```python
from build123d import *

# Parameters (mm, degrees)
F0_W        = 57.15
F0_H        = 50.8
F1_DEPTH    = 6.35
F2_W        = 13.208
F2_H        = 1.190625
F3_DEPTH    = 50.801
F4_SIZE     = 5.08
F5_W        = 3.4
F5_H        = 15
F6_DEPTH    = 18
F7_W        = 13.208
F7_H        = 1.5875
F8_DEPTH    = 57.151
F9_T1_DEPTH = 13.208
F9_T3_DEPTH = 13.208
F11_D       = 5
F12_DEPTH   = 36.676


# Not quite as in the source:
# - a fillet or chamfer that OpenCascade refuses, or shapes differently, is made with other operations: its cross-section is extruded or revolved along the edge and cut away or added


with BuildPart() as f1:
    # F0 (on Top) → F1 (new body)
    with BuildSketch(Plane.XY):
        Rectangle(F0_W, F0_H)
    extrude(amount=F1_DEPTH)

    # F2 (on face) → F3 (cut, through all)
    with BuildSketch(Plane.XZ.offset(25.4)):
        with Locations((-16.129, 5.7546875)):
            Rectangle(F2_W, F2_H)
        with Locations((16.129, 5.7546875)):
            Rectangle(F2_W, F2_H)
    extrude(amount=-F3_DEPTH, mode=Mode.SUBTRACT)

    # F4
    f4_edges = [f1.edges().sort_by_distance(p)[0] for p in [
        (-16.129, -25.4, 5.159375),
        (16.129, -25.4, 5.159375),
        (-16.129, 25.4, 5.159375),
        (16.129, 25.4, 5.159375),
    ]]
    chamfer(f4_edges, length=F4_SIZE)

    # F5 (on face) → F6 (join)
    with BuildSketch(Plane.XY.offset(6.35)):
        Rectangle(F5_W, F5_H)
        with Locations((6.4, 0)):
            Rectangle(F5_W, F5_H)
        with Locations((-6.4, 0)):
            Rectangle(F5_W, F5_H)
    extrude(amount=F6_DEPTH)

    # F7 (on face) → F8 (cut, through all)
    with BuildSketch(Plane.YZ.offset(28.575)):
        with Locations((-16.129, 5.55625)):
            Rectangle(F7_W, F7_H)
        with Locations((16.129, 5.55625)):
            Rectangle(F7_W, F7_H)
    extrude(amount=-F8_DEPTH, mode=Mode.SUBTRACT)

    # F9: chamfer of 5.08 on 4 edges, made by hand

    # F9_s2 → F9_t1 (cut)
    with BuildSketch(Plane.XZ.offset(-22.733)):
        Polygon((28.575, -0.3175), (23.495, 4.7625), (28.575, 4.7625), align=None)
        Polygon((-28.575, -0.3175), (-23.495, 4.7625), (-28.575, 4.7625), align=None)
    extrude(amount=F9_T1_DEPTH, mode=Mode.SUBTRACT)

    # F9_s4 → F9_t3 (cut)
    with BuildSketch(Plane.XZ.offset(9.525)):
        Polygon((28.575, -0.3175), (23.495, 4.7625), (28.575, 4.7625), align=None)
        Polygon((-28.575, -0.3175), (-23.495, 4.7625), (-28.575, 4.7625), align=None)
    extrude(amount=F9_T3_DEPTH, mode=Mode.SUBTRACT)

    # F11 (through all)
    with Locations(Plane.YZ.offset(8.1)):
        with Locations((0, 16.85)):
            Hole(F11_D / 2)

    # F10 (on face) → F12 (cut, through all)
    with BuildSketch(Plane.YZ.offset(8.1)):
        with BuildLine():
            Line((-7.5, 24.35), (-7.5, 16.85))
            ThreePointArc((-7.5, 16.85), (-5.3033008589, 22.1533008589), (0, 24.35))
            Line((0, 24.35), (-7.5, 24.35))
        make_face()
        with BuildLine():
            Line((7.5, 24.35), (0, 24.35))
            ThreePointArc((0, 24.35), (5.3033008589, 22.1533008589), (7.5, 16.85))
            Line((7.5, 16.85), (7.5, 24.35))
        make_face()
    extrude(amount=-F12_DEPTH, mode=Mode.SUBTRACT)


solid = f1.part
```
Geometry: final body of the model. Coordinates: model frame, mm. A direction names the side the tool comes from. Round coordinates to 2 decimals unless told otherwise and drop trailing zeros. Order: outer loops, then holes, each group sorted by start corner. A loop starts at its lowest first (then second) coordinate and runs counter-clockwise, first axis right, second up. Notation, with made-up numbers: M 64.25,3 L 122.25,3 A7 cw 122.25,8 Z; hole C 29,28.25 d2. An arc over 180 degrees is marked long. One line per item, written item: value.
(1) Pin query (flat end, axial travel): P1, Ø3, axis at x = -5, z = 19.5, coming from the +Y side; P2, Ø12, axis at y = 0, z = 14.5, coming from the +X side; P3, Ø4, axis at x = -15, y = -0.5, coming from the +Z side. Return the tip coordinate at first contact, or that it passes through.
Result sheet:
P1: y = 7.41
P2: x = 8.1
P3: z = 5.16
(2) Cut plane B-B (z = 9). Return the cut outline in (x, y).
Result sheet:
outline: M -8.1,-7.5 L -4.7,-7.5 L -4.7,7.5 L -8.1,7.5 Z; M -1.7,-7.5 L 1.7,-7.5 L 1.7,7.5 L -1.7,7.5 Z; M 4.7,-7.5 L 8.1,-7.5 L 8.1,7.5 L 4.7,7.5 Z
(3) Cut plane C-C (y = -6). Return the cut outline in (x, z) (3 decimals).
Result sheet:
outline: M -28.575,0 L 28.575,0 L 28.575,6.35 L 22.733,6.35 L 22.733,5.159 L 9.525,5.159 L 9.525,6.35 L 8.1,6.35 L 8.1,21.35 L 4.7,21.35 L 4.7,6.35 L 1.7,6.35 L 1.7,21.35 L -1.7,21.35 L -1.7,6.35 L -4.7,6.35 L -4.7,21.35 L -8.1,21.35 L -8.1,6.35 L -9.525,6.35 L -9.525,5.159 L -22.733,5.159 L -22.733,6.35 L -28.575,6.35 Z
(4) Pull-direction query (Y, two-part tool) for faces 1 (the flat face through (-9.525, 24, 4)), 2 (the flat face through (-26, -22.733, 4)), 3 (the flat face through (0, -7.5, 12)); classes: pulls with the +Y half, pulls with the -Y half, needs draft (parallel to the pull), parting line crosses it, or undercut.
Result sheet:
face 1: needs draft
face 2: undercut
face 3: pulls with the -Y half
(5) Reachability of faces 4 (the flat face through (-1.7, 0, 13)), 5 (the flat face through (0, -16, 4.762)), 6 (the flat face through (6, 7.5, 12)), 7 (the flat face through (-25.91, -16.04, 2.35)) from +Z, -Z, +X, -X, +Y, -Y: full face, straight path, thin tool, end or side. Return the list, or none.
Result sheet:
face 4: +Z, +Y, -Y
face 5: +Z, +X, -X
face 6: +Z, +X, -X, +Y
face 7: +Z, -X
(6) Line query: probe 1 along X at (y, z) = (4.5, 11); probe 2 along Z at (x, y) = (-6, 0); probe 3 along Z at (x, y) = (16.5, 10.5). Output: solid intervals per line, ascending. Write a range as [from, to].
Result sheet:
probe 1: [-8.1, -4.7], [-1.7, 1.7], [4.7, 8.1]
probe 2: [0, 14.35], [19.35, 24.35]
probe 3: [0, 4.76]
(7) Cut plane D-D (y = 0). Give the number of separate pieces and of enclosed holes in the cut face, and give its area (3 significant figures).
Result sheet:
separate pieces: 4
enclosed holes: 0
area: 464 mm2
